Source: CAD feature listing. Evaluate the final solid. Frame: model axes, mm. Face numbers are marked on the shaded views. A direction names the side the tool comes from. Give positions to 0.01 mm unless a question says otherwise; leave off trailing zeros. Write each question's results on one line, items separated by ' | '. Start each with the question number.
Item 1: Set-up query: the marked faces 1, 2 and 3. Return all of +Z, -Z, +X, -X, +Y, -Y with unobstructed straight access to the full face (end or side cutting, diameter ignored); none if empty.
Item 2: Line query: line 1 along X through (y, z) = (-40.5, -54); line 2 along X through (y, z) = (-20, 59); line 3 along X through (y, z) = (21.5, -6). Output: solid intervals per line, ascending.
Item 3: Mould query, pull axis Y, two halves, no side actions, for the marked faces 4, 5 and 6. Classes: released by +Y, released by -Y, zero draft, split by the parting line, or undercut.
Item 4: Contact query for flat-ended pins moving along their axis: pin 1 Ø1 at (x, z) = (-4.5, 25.5) entering from +Y; pin 2 Ø3 at (y, z) = (-2.5, 28.5) entering from -X; pin 3 Ø23 at (y, z) = (-32.5, 14.5) entering from +X. Output: stop coordinate, or through.
```python
from build123d import *

# Parameters (mm, degrees)
SKETCH_1_W             = 99
SKETCH_1_H             = 66
SKETCH_2_R             = 41
CUT_EXTRUDE_1_DEPTH    = 14.5
CUT_EXTRUDE_1_TAPER    = 2.29
FILLET_1_R             = 2
PATTERN_LINEAR_1_COUNT = 3
PATTERN_LINEAR_1_PITCH = 19
PATTERN_LINEAR_2_COUNT = 2
PATTERN_LINEAR_2_PITCH = 57
PATTERN_LINEAR_3_COUNT = 2
PATTERN_LINEAR_3_PITCH = 76
SKETCH_5_R             = 21
CUT_EXTRUDE_2_DEPTH    = 85.5
CHAMFER_1_SIZE         = 2
SKETCH_6_W             = 24
SKETCH_6_H             = 12
CUT_EXTRUDE_3_DEPTH    = 85.5


with BuildPart() as part:
    # Sketch 1 → Revolve 1 (revolve)
    with BuildSketch(Plane.XY):
        with Locations((30.45222636, 12.108822758)):
            Rectangle(SKETCH_1_W, SKETCH_1_H)
    revolve(axis=Axis((-19.04777364, -20.891177242, 0), (1, 0, 0)))

    # Sketch 2 → Cut-Extrude 1 (cut)
    with BuildSketch(Plane.ZY.offset(19.04777364)):
        with Locations((0, -20.891177242)):
            Circle(SKETCH_2_R)
    cut_extrude_1 = extrude(amount=-CUT_EXTRUDE_1_DEPTH, taper=CUT_EXTRUDE_1_TAPER, mode=Mode.SUBTRACT)

    # Mirror 1: Cut-Extrude 1 across plane
    add(cut_extrude_1.mirror(Plane.ZY.offset(-30.45222636)), mode=Mode.SUBTRACT)

    # Fillet 1
    fillet_1_edges = [part.edges().sort_by_distance(p)[0] for p in [
        (-4.54777364, -20.891177242, -40.420154632),
        (-19.04777364, -20.891177242, -41),
        (79.95222636, -20.891177242, -41),
        (65.45222636, -20.891177242, -40.420154632),
    ]]
    fillet(fillet_1_edges, radius=FILLET_1_R)

    # Sweep 1: sweep along a path in Sketch 4
    with BuildLine(Plane(origin=(72.394919545, 31.608822758, 0), x_dir=(0, 0, -1), z_dir=(1, 0, 0))) as sweep_1_path:
        CenterArc((0, -52.5), 52.5, 0, 360)
    # Sketch 3 → Sweep 1 (sweep, cut)
    with BuildSketch(Plane.XY):
        Polygon((64.509533174, 31.608822758), (72.394919545, 31.608822758), (76.522283745, 45.108822758), (60.382168975, 45.108822758), align=None)
    sweep_1 = sweep(path=sweep_1_path.line, mode=Mode.SUBTRACT)

    # Pattern Linear 1: Sweep 1 ×3
    with Locations(*[(-i * PATTERN_LINEAR_1_PITCH, 0, 0) for i in range(1, PATTERN_LINEAR_1_COUNT)]):
        add(sweep_1, mode=Mode.SUBTRACT)

    # Pattern Linear 2: Sweep 1 ×2
    with Locations(*[(-i * PATTERN_LINEAR_2_PITCH, 0, 0) for i in range(1, PATTERN_LINEAR_2_COUNT)]):
        add(sweep_1, mode=Mode.SUBTRACT)

    # Pattern Linear 3: Sweep 1 ×2
    with Locations(*[(-i * PATTERN_LINEAR_3_PITCH, 0, 0) for i in range(1, PATTERN_LINEAR_3_COUNT)]):
        add(sweep_1, mode=Mode.SUBTRACT)

    # Sketch 5 → Cut-Extrude 2 (cut, through all)
    with BuildSketch(Plane.ZY.offset(4.54777364)):
        with Locations((0, -20.891177242)):
            Circle(SKETCH_5_R)
    extrude(amount=-CUT_EXTRUDE_2_DEPTH, mode=Mode.SUBTRACT)

    # Chamfer 1
    chamfer_1_edges = [part.edges().sort_by_distance(p)[0] for p in [
        (65.45222636, -20.891177242, -21),
        (-4.54777364, -20.891177242, -21),
    ]]
    chamfer(chamfer_1_edges, length=CHAMFER_1_SIZE)

    # Sketch 6 → Cut-Extrude 3 (cut, through all)
    with BuildSketch(Plane(origin=(65.45222636, 0, 0), x_dir=(0, 0, -1), z_dir=(1, 0, 0))):
        with Locations((-12, -20.891177242)):
            Rectangle(SKETCH_6_W, SKETCH_6_H)
    extrude(amount=-CUT_EXTRUDE_3_DEPTH, mode=Mode.SUBTRACT)


solid = part.part
```
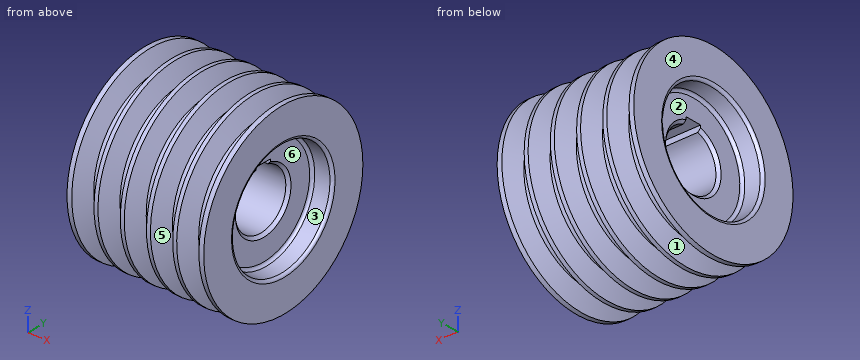
Evaluation:
1) face 1: none | face 2: -X | face 3: +X
2) line 1: x = -19.05 to -13, -2.09 to 6, 16.91 to 25, 35.91 to 44, 54.91 to 63, 73.91 to 79.95 | line 2: x = -19.05 to -13.48, -1.62 to 5.52, 17.38 to 24.52, 36.38 to 43.52, 55.38 to 62.52, 74.38 to 79.95 | line 3: x = -19.04 to 79.95
3) face 4: zero draft | face 5: split by the parting line | face 6: undercut
4) pin 1: stops at y = 25.27 | pin 2: stops at x = -4.55 | pin 3: stops at x = 65.45
